Verification items for the finished model (mm, model axes). A direction names the side the tool comes from. Round coordinates to 2 decimals unless told otherwise and drop trailing zeros. Order: outer loops, then holes, each group sorted by start corner. A loop starts at its lowest first (then second) coordinate and runs counter-clockwise, first axis right, second up. Notation, with made-up numbers: (-5.75, 37) -> (25.25, 37) arc R33 cw to (25.25, 72) -> close; hole circle Ø10 at (71, -23). An arc over 180 degrees is marked (long way). Put each result on its own line as item: value.
```python
from build123d import *

# Parameters (mm, degrees)
BOSS_EXTRUDE1_DEPTH = 10
BOSS_EXTRUDE2_DEPTH = 10
SKETCH3_R           = 12.5
BOSS_EXTRUDE3_DEPTH = 145
SKETCH4_R           = 2.5
BOSS_EXTRUDE4_DEPTH = 145
SKETCH5_R           = 15
BOSS_EXTRUDE5_DEPTH = 145
SKETCH6_R           = 12.5
BOSS_EXTRUDE6_DEPTH = 65
SKETCH7_W           = 150
SKETCH7_H           = 47.005771534
BOSS_EXTRUDE7_DEPTH = 15
SKETCH9_W           = 15
SKETCH9_H           = 47.005771534
BOSS_EXTRUDE8_DEPTH = 65
SKETCH10_W          = 150
SKETCH10_H          = 47.005771534
BOSS_EXTRUDE9_DEPTH = 15
SKETCH11_R          = 7.5
CUT_EXTRUDE1_DEPTH  = 15


with BuildPart() as part:
    # Sketch1 → Boss-Extrude1 (new body)
    with BuildSketch(Plane.XY):
        with BuildLine():
            Line((-190, 35), (190, 35))
            ThreePointArc((190, 35), (225, 0), (190, -35))
            Line((190, -35), (-190, -35))
            ThreePointArc((-190, -35), (-225, 0), (-190, 35))
        make_face()
    extrude(amount=BOSS_EXTRUDE1_DEPTH)



with BuildPart() as body_2:
    # Sketch2 → Boss-Extrude2 (new body)
    with BuildSketch(Plane.XY.offset(-120)):
        with BuildLine():
            Line((-190, 35), (190, 35))
            ThreePointArc((190, 35), (225, 0), (190, -35))
            Line((190, -35), (-190, -35))
            ThreePointArc((-190, -35), (-225, 0), (-190, 35))
        make_face()
    extrude(amount=-BOSS_EXTRUDE2_DEPTH)


with BuildPart() as part_1:
    add(part.part)

    add(body_2.part)  # Boss-Extrude3 merges body 2
    # Sketch3 → Boss-Extrude3 (add)
    with BuildSketch(Plane.XY.offset(10)):
        with Locations((-190, 0)):
            Circle(SKETCH3_R)
    extrude(amount=-BOSS_EXTRUDE3_DEPTH)

    # Sketch4 → Boss-Extrude4 (add)
    with BuildSketch(Plane.XY.offset(10)):
        with Locations((-125, 0)):
            Circle(SKETCH4_R)
    extrude(amount=-BOSS_EXTRUDE4_DEPTH)

    # Sketch5 → Boss-Extrude5 (add)
    with BuildSketch(Plane.XY.offset(10)):
        with Locations((190, 0)):
            Circle(SKETCH5_R)
    extrude(amount=-BOSS_EXTRUDE5_DEPTH)

    # Sketch6 → Boss-Extrude6 (add)
    with BuildSketch(Plane(origin=(190, 0, 0), x_dir=(0, 0, -1), z_dir=(1, 0, 0))):
        with Locations((60, 0)):
            Circle(SKETCH6_R)
    extrude(amount=BOSS_EXTRUDE6_DEPTH)

    # Sketch7 → Boss-Extrude7 (add)
    with BuildSketch(Plane(origin=(255, 0, 0), x_dir=(0, 0, -1), z_dir=(1, 0, 0))):
        with Locations((60, 0)):
            Rectangle(SKETCH7_W, SKETCH7_H)
    extrude(amount=BOSS_EXTRUDE7_DEPTH)

    # Sketch9 → Boss-Extrude8 (add)
    with BuildSketch(Plane(origin=(270, 0, 0), x_dir=(0, 0, -1), z_dir=(1, 0, 0))):
        with Locations((-7.5, 0)):
            Rectangle(SKETCH9_W, SKETCH9_H)
        with Locations((127.5, 0)):
            Rectangle(SKETCH9_W, SKETCH9_H)
    extrude(amount=BOSS_EXTRUDE8_DEPTH)

    # Sketch10 → Boss-Extrude9 (add)
    with BuildSketch(Plane(origin=(335, 0, 0), x_dir=(0, 0, -1), z_dir=(1, 0, 0))):
        with Locations((60, 0)):
            Rectangle(SKETCH10_W, SKETCH10_H)
    extrude(amount=BOSS_EXTRUDE9_DEPTH)

    # Sketch11 → Cut-Extrude1 (cut)
    with BuildSketch(Plane(origin=(350, 0, 0), x_dir=(0, 0, -1), z_dir=(1, 0, 0))):
        with Locations((60, 0)):
            Circle(SKETCH11_R)
    extrude(amount=-CUT_EXTRUDE1_DEPTH, mode=Mode.SUBTRACT)


solid = part_1.part
```
Item 1: Tool access check on faces 1 (the face through (-178.077, 3.755, -59.16)), 2 (the face through (302, 0, -120)), 3 (the face through (-178.077, 3.755, -132.465)). Record the directions out of +Z, -Z, +X, -X, +Y, -Y that give a thin tool (end or side, any length) a straight path to the whole face; none if there is none.
Geometry check:
face 1: none
face 2: +Y, -Y
face 3: -Z
Item 2: Sectioned sample at B-B, the plane x = -32. Record the boundary of the cut face in (y, z), then the cut area to 3 significant figures.
Geometry check:
outline: (-35, -130) -> (35, -130) -> (35, -120) -> (-35, -120) -> close; (-35, 0) -> (35, 0) -> (35, 10) -> (-35, 10) -> close
area: 1,400 mm2
Item 3: Release check for a two-part mould opening along X. For faces 4 (the face through (302, 0, 15)), 5 (the face through (3, 0, -130)), 6 (the face through (-224.99, -0.77, -124.93)) record: pulls with the +X half, pulls with the -X half, needs draft (parallel to the pull), parting line crosses it, or undercut.
Geometry check:
face 4: needs draft
face 5: undercut
face 6: pulls with the -X half
Item 4: Depth check by flat-ended pin: pin 1 Ø6 at (x, y) = (-79, -8) entering from -Z; pin 2 Ø10 at (y, z) = (25.5, -84) entering from -X; pin 3 Ø14 at (y, z) = (-3, -37.5) entering from -X. Enter the tip coordinate at first touch or a pass-through.
Geometry check:
pin 1: z = -130
pin 2: x = 255
pin 3: x = -202.5
Item 5: Sectioned sample at A-A, the plane z = -60. Record the boundary of the cut face in (x, y).
Geometry check:
outline: circle Ø25 at (-190, 0); circle Ø5 at (-125, 0); (198.29, -12.5) -> (255, -12.5) -> (255, -23.5) -> (270, -23.5) -> (270, 23.5) -> (255, 23.5) -> (255, 12.5) -> (198.29, 12.5) arc R15 ccw (long way) to start; (335, -23.5) -> (350, -23.5) -> (350, -7.5) -> (335, -7.5) -> close; (335, 7.5) -> (350, 7.5) -> (350, 23.5) -> (335, 23.5) -> close
Item 6: Material ranges on line 1 along Z through (x, y) = (-23, -7); line 2 along Y through (x, z) = (340, -60); line 3 along X through (y, z) = (-2, -42), recorded low to high.
Geometry check:
line 1: -130 to -120, 0 to 10
line 2: -23.5 to -7.5, 7.5 to 23.5
line 3: -202.34 to -177.66, -126.5 to -123.5, 175.13 to 204.87, 255 to 270, 335 to 350
